Read the model definition and answer for the solid it produces. Units are mm, in the model's axes. A direction names the side the tool comes from. Give positions to 0.01 mm unless a question says otherwise; leave off trailing zeros. Write each loop counter-clockwise with the first axis right and the second up, starting at its lowest first coordinate (ties: lowest second). Pieces come first, ordered by that corner, then holes.
```python
from build123d import *

# Parameters (mm, degrees)
SKETCH3_W                                       = 57.15
SKETCH3_H                                       = 50
BOSS_EXTRUDE1_DEPTH                             = 8
SKETCH3_3_R                                     = 1.5
SKETCH3_3_R_2                                   = 8
CUT_EXTRUDE2_DEPTH                              = 10
SKETCH4_R                                       = 18.5
CUT_EXTRUDE3_DEPTH                              = 4
BOSS_EXTRUDE2_DEPTH                             = 15
BOSS_EXTRUDE2_DEPTH_BACK                        = 23
SKETCH6_W                                       = 80
SKETCH6_H                                       = 5
CSK_FOR_M3_FLAT_HEAD_MACHINE_SCREW1_D           = 3.4
CSK_FOR_M3_FLAT_HEAD_MACHINE_SCREW1_CSINK_D     = 6.3
CSK_FOR_M3_FLAT_HEAD_MACHINE_SCREW1_CSINK_ANGLE = 90
CUT_EXTRUDE8_REACH                              = 66.452
SKETCH14_W                                      = 15.24
SKETCH14_H                                      = 38
CUT_EXTRUDE8_DIRECTION_2_DEPTH                  = 45
BOSS_EXTRUDE5_START                             = 3.175
SKETCH15_W                                      = 64.76
SKETCH15_H                                      = 38
SKETCH15_R                                      = 1.7
BOSS_EXTRUDE5_DEPTH                             = 3.175


with BuildPart() as part:
    # Sketch3 → Boss-Extrude1 (new body)
    with BuildSketch(Plane.XY):
        with Locations((0, 25)):
            Rectangle(SKETCH3_W, SKETCH3_H)
    extrude(amount=BOSS_EXTRUDE1_DEPTH)

    # Sketch3<3> → Cut-Extrude2 (cut)
    with BuildSketch(Plane.XY):
        with Locations(Location((-7.75, 38.423393759, 0), (0, 0, 180))):
            Circle(SKETCH3_3_R)
        with Locations(Location((7.75, 38.423393759, 0), (0, 0, 180))):
            Circle(SKETCH3_3_R)
        with Locations(Location((-7.75, 11.576606241, 0), (0, 0, 180))):
            Circle(SKETCH3_3_R)
        with Locations(Location((7.75, 11.576606241, 0), (0, 0, 180))):
            Circle(SKETCH3_3_R)
        with Locations(Location((15.5, 25, 0), (0, 0, 180))):
            Circle(SKETCH3_3_R)
        with Locations(Location((6.062177825, 28.499999999, 0), (0, 0, 180))):
            Circle(SKETCH3_3_R_2)
    extrude(amount=CUT_EXTRUDE2_DEPTH, mode=Mode.SUBTRACT)

    # Sketch4 → Cut-Extrude3 (cut)
    with BuildSketch(Plane.XY.offset(8)):
        with Locations((0, 25)):
            Circle(SKETCH4_R)
    extrude(amount=-CUT_EXTRUDE3_DEPTH, mode=Mode.SUBTRACT)

    # Sketch6 → Boss-Extrude2 (add, two sides: drawn at the far end of the back side and taken through both)
    with BuildSketch(Plane.XY.offset(8).offset(-BOSS_EXTRUDE2_DEPTH_BACK)):
        with Locations((0, 2.5)):
            Rectangle(SKETCH6_W, SKETCH6_H)
    extrude(amount=BOSS_EXTRUDE2_DEPTH + BOSS_EXTRUDE2_DEPTH_BACK)

    # CSK for M3 Flat Head Machine Screw1 (through all)
    with Locations(Plane(origin=(0, 5, 0), x_dir=(1, 0, 0), z_dir=(0, 1, 0))):
        with Locations((-32.5, 7.5), (-32.5, -15.5), (32.5, -15.5), (32.5, 7.5)):
            CounterSinkHole(CSK_FOR_M3_FLAT_HEAD_MACHINE_SCREW1_D / 2, CSK_FOR_M3_FLAT_HEAD_MACHINE_SCREW1_CSINK_D / 2, counter_sink_angle=CSK_FOR_M3_FLAT_HEAD_MACHINE_SCREW1_CSINK_ANGLE)

    # Sketch14 → Cut-Extrude8 (cut, up to next)
    with BuildSketch(Plane(origin=(0, 5, 0), x_dir=(1, 0, 0), z_dir=(0, 1, 0)), mode=Mode.PRIVATE) as cut_extrude8_sk1:
        with Locations((-32.38, -4)):
            Rectangle(SKETCH14_W, SKETCH14_H)
    cut_extrude8_tool1 = extrude(cut_extrude8_sk1.sketch, amount=-CUT_EXTRUDE8_REACH, mode=Mode.PRIVATE) & part.part
    add(cut_extrude8_tool1.solids().sort_by_distance((-32.38, 5, 4))[0], mode=Mode.SUBTRACT)

    # Sketch14 → Cut-Extrude8 direction 2 (cut)
    with BuildSketch(Plane(origin=(0, 5, 0), x_dir=(1, 0, 0), z_dir=(0, 1, 0))):
        with Locations((-32.38, -4)):
            Rectangle(SKETCH14_W, SKETCH14_H)
    extrude(amount=CUT_EXTRUDE8_DIRECTION_2_DEPTH, mode=Mode.SUBTRACT)

    # Sketch15 → Boss-Extrude5 (add)
    with BuildSketch(Plane.XZ.offset(BOSS_EXTRUDE5_START)):
        with Locations((7.62, 4)):
            Rectangle(SKETCH15_W, SKETCH15_H)
        with Locations(Location((32.5, 15.5, 0), (0, 0, 90))):
            Circle(SKETCH15_R, mode=Mode.SUBTRACT)
        with Locations(Location((32.5, -7.5, 0), (0, 0, 90))):
            Circle(SKETCH15_R, mode=Mode.SUBTRACT)
    extrude(amount=-BOSS_EXTRUDE5_DEPTH)


solid = part.part
```
Item 1: Section A-A (z = -7.5) is taken. Write down the section's boundary in (x, y) (3 decimals), and give its area (3 significant figures).
Result set:
outline: (-24.76, -3.175) - (30.8, -3.175) - (30.8, 3.55) - (29.35, 5) - (-24.76, 5) - close; (34.2, -3.175) - (40, -3.175) - (40, 5) - (35.65, 5) - (34.2, 3.55) - close
area: 500 mm2
Item 2: Each of these flat-tipped pins is pushed along its axis until it touches: pin 1 Ø12 at (x, y) = (-15, 16) entering from +Z; pin 2 Ø1.5 at (x, z) = (8.5, -8.5) entering from +Y; pin 3 Ø5.5 at (x, z) = (32.5, -7.5) entering from +Y; pin 4 Ø1.8 at (x, y) = (7.75, 38.42) entering from -Z. Where does it stop, or does it pass through?
Result set:
pin 1: stops at z = 8
pin 2: stops at y = 5
pin 3: stops at y = 4.6
pin 4: passes through
Item 3: Section D-D (x = -7.75) is taken. Write down the section's boundary in (y, z) (3 decimals), and give its area (3 significant figures).
Result set:
outline: (-3.175, -15) - (5, -15) - (5, 0) - (10.077, 0) - (10.077, 4) - (8.202, 4) - (8.202, 8) - (5, 8) - (5, 23) - (-3.175, 23) - close; (13.077, 0) - (36.923, 0) - (36.923, 4) - (13.077, 4) - close; (39.923, 0) - (50, 0) - (50, 8) - (41.798, 8) - (41.798, 4) - (39.923, 4) - close
area: 512 mm2
Item 4: Section C-C (y = 32) is taken. Write down the section's boundary in (x, z) (3 decimals), and give its area (3 significant figures).
Result set:
outline: (-24.76, 0) - (-1.132, 0) - (-1.132, 4) - (-17.125, 4) - (-17.125, 8) - (-24.76, 8) - close; (13.256, 0) - (28.575, 0) - (28.575, 8) - (17.125, 8) - (17.125, 4) - (13.256, 4) - close
area: 232 mm2
Item 5: Find the intervals of material crossed by line 1 along Y through (x, z) = (-7.75, 2.1) (3 decimals); line 2 along Y through (x, z) = (7.75, 3) (3 decimals); line 3 along Z through (x, y) = (-19, 9), in increasing order.
Result set:
line 1: y = -3.175 to 10.077, 13.077 to 36.923, 39.923 to 50
line 2: y = -3.175 to 10.077, 13.077 to 20.68, 36.32 to 36.923, 39.923 to 50
line 3: z = 0 to 8
Item 6: Determine the mould class of faces 1 (the flat face through (7, 1, 23)), 2 (the cylindrical face through (9.25, 11.51, 1.97)), 3 (the cylindrical face through (31.87, -0.61, -5.92)) for opening direction Z: pulls with the +Z half, pulls with the -Z half, needs draft (parallel to the pull), parting line crosses it, or undercut.
Result set:
face 1: pulls with the +Z half
face 2: needs draft
face 3: undercut
Item 7: Section B-B (x = 4) is taken. Write down the section's boundary in (y, z) (3 decimals), and give its area (3 significant figures).
Result set:
outline: (-3.175, -15) - (5, -15) - (5, 0) - (20.77, 0) - (20.77, 4) - (6.938, 4) - (6.938, 8) - (5, 8) - (5, 23) - (-3.175, 23) - close; (36.23, 0) - (50, 0) - (50, 8) - (43.062, 8) - (43.062, 4) - (36.23, 4) - close
area: 464 mm2
Item 8: Which of the six approach directions +Z, -Z, +X, -X, +Y, -Y give full straight-line access (tool end or side, diameter ignored) to faces 4 (the flat face through (-4, 28, 0)), 5 (the flat face through (28.575, 27, 4)), 6 (the cylindrical face through (-6.644, 10.563, 1.972)), 7 (the flat face through (-24.76, 13, 3)), 8 (the flat face through (7, 43, 8))?
Result set:
face 4: -Z, +X, -X, +Y
face 5: +Z, -Z, +X, +Y
face 6: +Z, -Z
face 7: +Z, -Z, -X, +Y, -Y
face 8: +Z, +X, -X, +Y
